The listing builds one solid part. Answer for the finished solid, in the listing's coordinates (mm). Face numbers are marked on the shaded views. A direction names the side the tool comes from. Round coordinates to 2 decimals unless told otherwise and drop trailing zeros. Write each loop counter-clockwise with the first axis right and the second up, starting at its lowest first coordinate (ties: lowest second). Pieces come first, ordered by that corner, then holes. Notation, with made-up numbers: (-9, 87) - (50, 87) arc R24 cw to (50, 102) - close; hole circle Ø6 at (-8, 1.5). An arc over 180 degrees is marked (long way). Return JSON: item names as keys, results as strings. Group by question number.
(1) Which of the six approach directions +Z, -Z, +X, -X, +Y, -Y give full straight-line access (tool end or side, diameter ignored) to the marked faces 3 and 4?
(2) Section A-A, the plane z = 0 is taken. Write down the section's boundary in (x, y), then the cut area to 3 significant figures.
(3) Determine the mould class of the marked faces 1 and 2 for opening direction Z: +Z half, -Z half, draft (parallel to the pull), parting line (faces both ways), or undercut.
(4) Section B-B, the plane y = -0.75 is taken. Write down the section's boundary in (x, z), then the cut area to 3 significant figures.
(5) Find the intervals of material crossed by line 1 along Y through (x, z) = (-0.5, 0); line 2 along Y through (x, z) = (0.75, 0); line 3 along Y through (x, z) = (1.75, -4), in increasing order. Write a range as [from, to].
(6) Each of these flat-tipped pins is pushed along its axis until it touches: pin 1 (4 mm diameter, centred on x = -1, z = 7, fed in from +Y); pin 2 (1.5 mm diameter, centred on x = 0.5, y = -4, fed in from -Z); pin 3 (5 mm diameter, centred on y = 0, z = 0, fed in from +X) (3 decimals). Where does it stop, or does it pass through?
```python
from build123d import *

# Parameters (mm, degrees)
BASPROSKE_W      = 5
BASPROSKE_H      = 12
TOOTHCUT_DEPTH   = 18.691806013
TEETHCUTS_COUNT  = 10
TEETHCUTS_ANGLE  = 324
HUBNEAONESKE_R   = 6
HUBNEARONE_DEPTH = 3.0000508
BORSKE_R         = 3
BORE_DEPTH       = 8.0000508


with BuildPart() as part:
    # BasProSke → Base-Revolve (revolve)
    with BuildSketch(Plane(origin=(0, 0, 0), x_dir=(1, 0, 0), z_dir=(0, 1, 0)), mode=Mode.PRIVATE) as base_revolve_sk:
        with Locations((2.5, 6)):
            Rectangle(BASPROSKE_W, BASPROSKE_H)
    revolve(base_revolve_sk.sketch.rotate(Axis((-10, 0, 0), (1, 0, 0)), 180), axis=Axis((-10, 0, 0), (1, 0, 0)))

    # TooCutSke → ToothCut (cut, through all)
    with BuildSketch(Plane(origin=(0, 0, 0), x_dir=(0, 0, -1), z_dir=(1, 0, 0))):
        with BuildLine():
            ThreePointArc((1.173662691, 7.406586048), (0, 7.499), (-1.173662691, 7.406586048))
            ThreePointArc((-1.173662691, 7.406586048), (-1.668191438, 9.834565786), (-3.497907776, 11.50542856))
            ThreePointArc((-3.497907776, 11.50542856), (0, 12.0254), (3.497907776, 11.50542856))
            ThreePointArc((3.497907776, 11.50542856), (1.668191438, 9.834565786), (1.173662691, 7.406586048))
        make_face()
    toothcut = extrude(amount=TOOTHCUT_DEPTH, mode=Mode.SUBTRACT)

    # TeethCuts: ToothCut ×10 about axis
    teethcuts_axis = Axis((-10, 0, 0), (1, 0, 0))
    for i in range(1, TEETHCUTS_COUNT):
        add(toothcut.rotate(teethcuts_axis, i * TEETHCUTS_ANGLE / (TEETHCUTS_COUNT - 1)), mode=Mode.SUBTRACT)

    # HubNeaOneSke → HubNearOne (add)
    with BuildSketch(Plane.ZY):
        with Locations(Location((0, 0, 0), (0, 0, 180))):
            Circle(HUBNEAONESKE_R)
    extrude(amount=HUBNEARONE_DEPTH)

    # BorSke → Bore (cut, symmetric)
    with BuildSketch(Plane(origin=(0, 0, 0), x_dir=(0, 0, -1), z_dir=(1, 0, 0))):
        with Locations(Location((0, 0, 0), (0, 0, 180))):
            Circle(BORSKE_R)
    extrude(amount=BORE_DEPTH, both=True, mode=Mode.SUBTRACT)


solid = part.part
```
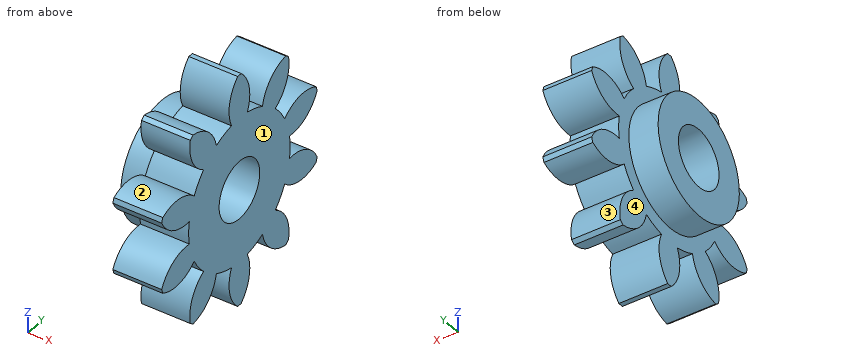
Working result:
{
 "1": {"face 3": "+X, -X, +Y", "face 4": "-X"},
 "2": {"outline": "(-3, -6) - (0, -6) - (0, -7.5) - (5, -7.5) - (5, -3) - (-3, -3) - close; (-3, 3) - (5, 3) - (5, 7.5) - (0, 7.5) - (0, 6) - (-3, 6) - close", "area": "63.0 mm^2"},
 "3": {"face 1": "draft", "face 2": "undercut"},
 "4": {"outline": "(-3, -5.95) - (0, -5.95) - (0, -11.45) - (5, -11.45) - (5, -2.9) - (-3, -2.9) - close; (-3, 2.9) - (5, 2.9) - (5, 11.45) - (0, 11.45) - (0, 5.95) - (-3, 5.95) - close", "area": "104 mm^2"},
 "5": {"line 1": "y = [-6, -3], [3, 6]", "line 2": "y = [-7.5, -3], [3, 7.5]", "line 3": "y = [-11.24, -7.53], [-6.34, 6.34], [7.53, 11.24]"},
 "6": {"pin 1": "stops at y = 7.33", "pin 2": "stops at z = -8.95", "pin 3": "passes through"}
}
